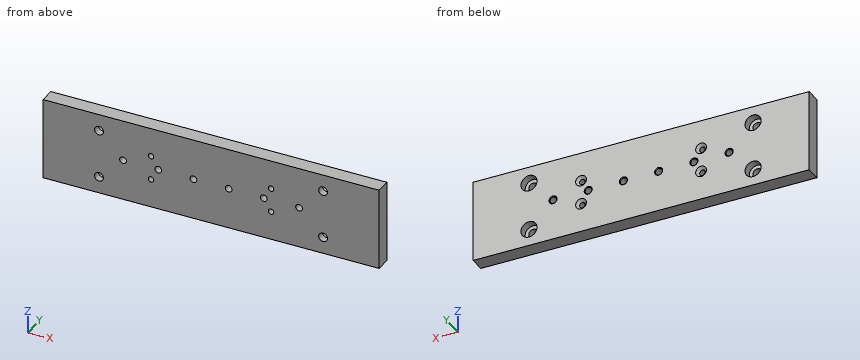
from build123d import *

# Parameters (mm, degrees)
SKETCH1_W                       = 210
SKETCH1_H                       = 50.8
BOSS_EXTRUDE1_DEPTH             = 9.525
CSK_FOR_M3_SFHCS1_D             = 3.4
CSK_FOR_M3_SFHCS1_CSINK_D       = 6.72
CSK_FOR_M3_SFHCS1_CSINK_ANGLE   = 90
CBORE_FOR_M5_SHCS1_D            = 5.5
CBORE_FOR_M5_SHCS1_CBORE_D      = 10
CBORE_FOR_M5_SHCS1_CBORE_DEPTH  = 5
M5X0_8_TAPPED_HOLE1_D           = 4.2
M5X0_8_TAPPED_HOLE1_CSINK_D     = 5.05
M5X0_8_TAPPED_HOLE1_CSINK_ANGLE = 90


with BuildPart() as part:
    # Sketch1 → Boss-Extrude1 (new body)
    with BuildSketch(Plane(origin=(0, 0, 0), x_dir=(1, 0, 0), z_dir=(0, 1, 0))):
        Rectangle(SKETCH1_W, SKETCH1_H)
    extrude(amount=BOSS_EXTRUDE1_DEPTH)

    # CSK for M3 SFHCS1 (through all)
    with Locations(Plane(origin=(0, 9.525, 0), x_dir=(1, 0, 0), z_dir=(0, 1, 0))):
        with Locations((-37.5, 7.5), (-37.5, -7.5), (37.5, -7.5), (37.5, 7.5)):
            CounterSinkHole(CSK_FOR_M3_SFHCS1_D / 2, CSK_FOR_M3_SFHCS1_CSINK_D / 2, counter_sink_angle=CSK_FOR_M3_SFHCS1_CSINK_ANGLE)

    # CBORE for M5 SHCS1 (through all)
    with Locations(Plane(origin=(0, 9.525, 0), x_dir=(1, 0, 0), z_dir=(0, 1, 0))):
        with Locations((-70, -15), (-70, 15)):
            cbore_for_m5_shcs1 = CounterBoreHole(CBORE_FOR_M5_SHCS1_D / 2, CBORE_FOR_M5_SHCS1_CBORE_D / 2, CBORE_FOR_M5_SHCS1_CBORE_DEPTH)

    # Mirror1: CBORE for M5 SHCS1 across plane
    add(cbore_for_m5_shcs1.mirror(Plane(origin=(0, 0, 0), x_dir=(0, 0, 1), z_dir=(1, 0, 0))), mode=Mode.SUBTRACT)

    # M5x0.8 Tapped Hole1 (through all)
    with Locations(Plane(origin=(0, 9.525, 0), x_dir=(1, 0, 0), z_dir=(0, 1, 0))):
        with Locations((-55, 0), (-33, 0), (-11, 0), (11, 0), (33, 0), (55, 0)):
            CounterSinkHole(M5X0_8_TAPPED_HOLE1_D / 2, M5X0_8_TAPPED_HOLE1_CSINK_D / 2, counter_sink_angle=M5X0_8_TAPPED_HOLE1_CSINK_ANGLE)


solid = part.part
Could you check a few things on this model? Use its own coordinates, in mm. Give positions to 0.01 mm unless a question says otherwise; leave off trailing zeros. Write each loop counter-clockwise with the first axis right and the second up, starting at its lowest first coordinate (ties: lowest second). Pieces come first, ordered by that corner, then holes. Notation, with made-up numbers: (24.5, 24) -> (33.5, 24) arc R19 cw to (33.5, 48) -> close; hole circle Ø6 at (9, 42.25). An arc over 180 degrees is marked (long way). Answer as a JSON object with one key per item and string values.
Q1. Will these pins go through, and if not, where does the flat tip stop? pin 1 Ø2.5 at (x, z) = (55, 0) entering from -Y; pin 2 Ø5 at (x, z) = (-11, 0) entering from +Y; pin 3 Ø5 at (x, z) = (70, 13.5) entering from +Y (3 decimals); pin 4 Ø5.5 at (x, z) = (-37.5, -7.5) entering from +Y (3 decimals).
Taken from the geometry:
{"pin 1": "passes through", "pin 2": "stops at y = 9.5", "pin 3": "stops at y = 4.525", "pin 4": "stops at y = 8.915"}
Q2. Suppose I cut it at C-C on y = 1.75. Count the separate pieces of the cut face and the enclosed holes in it, then the cut area to 3 significant figures.
Taken from the geometry:
{"separate pieces": "1", "enclosed holes": "14", "area": "10,500 mm²"}
Q3. Suppose I cut it at A-A on x = -55. Write out the boundary of the cut face in (y, z) (3 decimals).
Taken from the geometry:
{"outline": "(0, -25.4) -> (9.525, -25.4) -> (9.525, -2.525) -> (9.1, -2.1) -> (0, -2.1) -> close; (0, 2.1) -> (9.1, 2.1) -> (9.525, 2.525) -> (9.525, 25.4) -> (0, 25.4) -> close"}
Q4. Suppose I cut it at B-B on z = -15. Write out the boundary of the cut face in (x, y) (3 decimals).
Taken from the geometry:
{"outline": "(-105, 0) -> (-72.75, 0) -> (-72.75, 4.525) -> (-75, 4.525) -> (-75, 9.525) -> (-105, 9.525) -> close; (-67.25, 0) -> (67.25, 0) -> (67.25, 4.525) -> (65, 4.525) -> (65, 9.525) -> (-65, 9.525) -> (-65, 4.525) -> (-67.25, 4.525) -> close; (72.75, 0) -> (105, 0) -> (105, 9.525) -> (75, 9.525) -> (75, 4.525) -> (72.75, 4.525) -> close"}
Q5. Please list where these lines run through material, in increasing order: L1, parallel to Z at x = -70, y = 2.25; L2, parallel to X at y = 2.6, z = -15; L3, parallel to Z at x = -70, y = 7.3.
Taken from the geometry:
{"L1": "z = -25.4 to -17.75, -12.25 to 12.25, 17.75 to 25.4", "L2": "x = -105 to -72.75, -67.25 to 67.25, 72.75 to 105", "L3": "z = -25.4 to -20, -10 to 10, 20 to 25.4"}
